```python
from build123d import *

# Parameters (mm, degrees)
PROFILE_SKETCH_R              = 10
PROFILE_SKETCH_R_2            = 5
CYLINDER_EXTRUDE_DEPTH        = 26
LIP_RING_SKETCH_R             = 7
LIP_RING_SKETCH_R_2           = 5
BOTTOM_LIP_RING_EXTRUDE_DEPTH = 1
BOTTOM_RING_FILLET_R          = 1
TOP_START                     = -27
SKETCH2_2_R                   = 7
SKETCH2_2_R_2                 = 5
TOP_LIP_RING_EXTRUDE_DEPTH    = 1
TOP_RING_FILLET_R             = 1


with BuildPart() as part:
    # Profile Sketch → Cylinder Extrude (new body)
    with BuildSketch(Plane(origin=(0, 0, 0), x_dir=(1, 0, 0), z_dir=(0, 1, 0))):
        with Locations(Location((0, 0, 0), (0, 0, 90))):
            Circle(PROFILE_SKETCH_R)
        with Locations(Location((0, 0, 0), (0, 0, 90))):
            Circle(PROFILE_SKETCH_R_2, mode=Mode.SUBTRACT)
    extrude(amount=CYLINDER_EXTRUDE_DEPTH)

    # Lip Ring Sketch → Bottom Lip Ring Extrude (add)
    with BuildSketch(Plane(origin=(0, 26, 0), x_dir=(1, 0, 0), z_dir=(0, 1, 0))):
        with Locations(Location((0, 0, 0), (0, 0, 270))):
            Circle(LIP_RING_SKETCH_R)
        with Locations(Location((0, 0, 0), (0, 0, 90))):
            Circle(LIP_RING_SKETCH_R_2, mode=Mode.SUBTRACT)
    extrude(amount=BOTTOM_LIP_RING_EXTRUDE_DEPTH)

    # Bottom Ring Fillet
    bottom_ring_fillet_edges = [part.edges().sort_by_distance(p)[0] for p in [
        (0, 27, -7),
        (0, 27, 5),
    ]]
    fillet(bottom_ring_fillet_edges, radius=BOTTOM_RING_FILLET_R - 0.0001)  # a hair under: the kernel refuses the full size

    # Sketch2<2> → Top Lip Ring Extrude (add)
    with BuildSketch(Plane(origin=(0, 26, 0), x_dir=(1, 0, 0), z_dir=(0, 1, 0)).offset(TOP_START)):
        with Locations(Location((0, 0, 0), (0, 0, 270))):
            Circle(SKETCH2_2_R)
        with Locations(Location((0, 0, 0), (0, 0, 90))):
            Circle(SKETCH2_2_R_2, mode=Mode.SUBTRACT)
    extrude(amount=TOP_LIP_RING_EXTRUDE_DEPTH)

    # Top Ring Fillet
    top_ring_fillet_edges = [part.edges().sort_by_distance(p)[0] for p in [
        (0, -1, -7),
        (0, -1, 5),
    ]]
    fillet(top_ring_fillet_edges, radius=TOP_RING_FILLET_R - 0.0001)  # a hair under: the kernel refuses the full size


solid = part.part
```
Geometry check sheet. Reference: the model listing, model coordinates, mm. Round coordinates to 2 decimals unless told otherwise and drop trailing zeros. Order: outer loops, then holes, each group sorted by start corner. A loop starts at its lowest first (then second) coordinate and runs counter-clockwise, first axis right, second up. Notation, with made-up numbers: (21, 15) -> (39, 15) arc R5 ccw to (39, 23) -> close; hole circle Ø6 at (-7.5, 5). An arc over 180 degrees is marked (long way). Return JSON: item names as keys, results as strings. Group by question number.
Q1. Section check C-C, the plane y = 15. Record the boundary of the cut face in (x, z).
Q2. Gauge pin test, flat ends, axial feed: pin 1 (8 mm diameter, centred on x = -0.5, z = -1.5, fed in from -Y); pin 2 (6 mm diameter, centred on x = -5, y = 10.5, fed in from -Z); pin 3 (6 mm diameter, centred on x = -1.5, z = 1, fed in from +Y); pin 4 (1 mm diameter, centred on x = 5.5, y = 15.5, fed in from +Z). Record the tip position at first contact, or that the pin passes through.
Q3. Release check for a two-part mould opening along X. For faces 1 (the cylindrical face through (4.88, 12.82, 1.08)), 2 (the cylindrical face through (9.76, 12.82, 2.17)), 3 (the flat face through (-7, 26, -2)) record: released by +X, released by -X, zero draft, split by the parting line, or undercut.
Q4. Material ranges on probe 1 along X at (y, z) = (8.75, 0); probe 2 along Y at (x, z) = (-7.25, -2.75); probe 3 along X at (y, z) = (17, -3.5), recorded low to high. Write a range as from..to.
Q5. Section check D-D, the plane z = -7.5. Record the boundary of the cut face in (x, y), plus the area to 3 significant figures.
Numbers:
{
 "1": {"outline": "circle Ø20 at (0, 0); hole circle Ø10 at (0, 0)"},
 "2": {"pin 1": "y = -0.91", "pin 2": "z = -9.8", "pin 3": "through", "pin 4": "z = 8.66"},
 "3": {"face 1": "undercut", "face 2": "split by the parting line", "face 3": "zero draft"},
 "4": {"probe 1": "-10..-5, 5..10", "probe 2": "0..26", "probe 3": "-9.37..-3.57, 3.57..9.37"},
 "5": {"outline": "(-6.61, 0) -> (6.61, 0) -> (6.61, 26) -> (-6.61, 26) -> close", "area": "344 mm^2"}
}
